Here's the drawing with two shaded views (mm, measured from the low corner). I have some questions. Give positions to 0.01 mm unless a question says otherwise; leave off trailing zeros. Put each result on its own line as item: value.
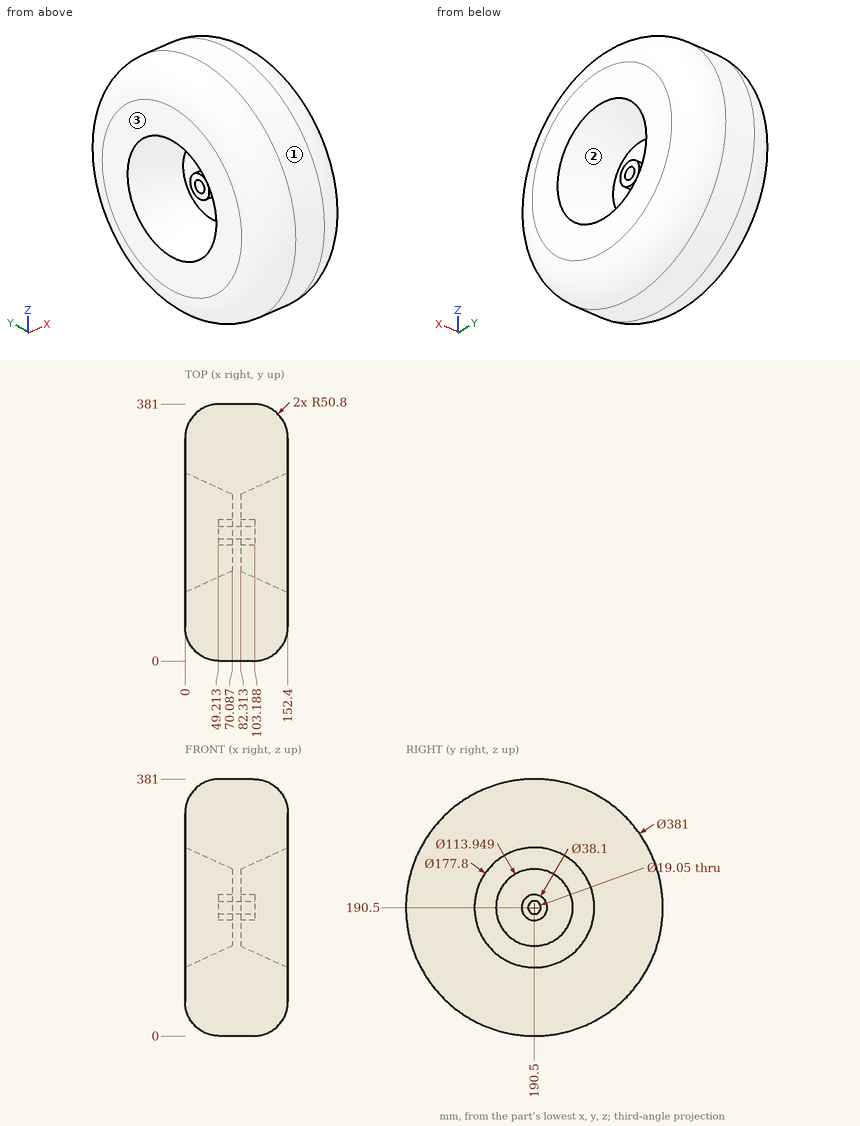
1. I'm going to push flat-ended pins straight in: pin 1 (10 mm diameter, centred on y = 333.5, z = 153.5, fed in from +X); pin 2 (6 mm diameter, centred on x = 39, y = 317, fed in from +Z); pin 3 (4 mm diameter, centred on x = 92, z = 287, fed in from -Y). Where does each tip first touch, or does it pass through?
Recorded:
pin 1: stops at x = 152.31
pin 2: stops at z = 333.87
pin 3: stops at y = 25.09
2. Thinking about a two-plate mould opening in Y: for the marked faces 1, 2 and 3, which applies, pulls with the +Y half, pulls with the -Y half, needs draft (parallel to the pull), parting line crosses it, or undercut?
Recorded:
face 1: parting line crosses it
face 2: undercut
face 3: needs draft
3. I need wall thicknesses on line 1 (Z direction, x = 77, y = 190); line 2 (Z direction, x = 67, y = 190) (1 decimal); line 3 (Y direction, x = 88, z = 190) (1 decimal). Which ranges of each line are inside material? Lowest first, please.
Recorded:
line 1: z = 0 to 180.99, 200.01 to 381
line 2: z = 0 to 132.1, 171.5 to 181, 200 to 209.5, 248.9 to 381
line 3: y = 0 to 130.9, 171.5 to 181, 200 to 209.5, 250.1 to 381
